Build history of the part. All positions in model axes, mm. A direction names the side the tool comes from. Round coordinates to 2 decimals unless told otherwise and drop trailing zeros. Write each loop counter-clockwise with the first axis right and the second up, starting at its lowest first coordinate (ties: lowest second). Pieces come first, ordered by that corner, then holes.
Item 1: Band-saw the part on C-C, the plane x = -3. Write the cut outline in (y, z), then the cut area to 3 significant figures.
Item 2: Wall check: probe 1 along Y at (x, z) = (1.75, 5.25); probe 2 along Y at (x, z) = (-1, 2); probe 3 along X at (y, z) = (3, -2.25). Give the ranges that are in metal, low to high.
Item 3: Band-saw the part on B-B, the plane x = 0. Write the cut outline in (y, z).
Item 4: 3-axis set-ups, long thin cutter, end or side, ignore diameter. For faces 4 (the cylindrical face through (0, 1.1, 2.7)), 5 (the flat face through (-5.5, 16, 0)): which of +Z, -Z, +X, -X, +Y, -Y reach the whole face in a straight line?
Item 5: Band-saw the part on A-A, the plane y = 4. Write the cut outline in (x, z) (1 decimal).
Item 6: Mould opens along X. For faces 1 (the flat face through (0, 5, 1.7)), 2 (the flat face through (0, 16, -5.5)), 3 (the flat face through (5.5, 16, 0)) say: +X half, -X half, draft (parallel to the pull), parting line (faces both ways), or undercut.
Item 7: Drop flat-ended pins along their axis: pin 1 Ø1 at (x, y) = (-3, 10.5) entering from +Z; pin 2 Ø1 at (x, z) = (1.5, -0.5) entering from -Y; pin 3 Ø1.1 at (y, z) = (3, 0.5) entering from -X. Give the stop position or say it passes through.
Autodesk Inventor part; units mm, degrees
ref_plane "YZ Plane" through (0, 0, 0) normal (1, 0, 0) x (0, 1, 0)
ref_plane "XZ Plane" through (0, 0, 0) normal (0, 1, 0) x (-1, 0, 0)
ref_plane "XY Plane" through (0, 0, 0) normal (0, 0, 1) x (1, 0, 0)
sketch "Sketch1" plane through (0, 0, 0) normal (0, 1, 0) x (-1, 0, 0)
  line L0 (14.5, -14.5) -> (-14.5, -14.5)
  line L1 (-14.5, -14.5) -> (-14.5, 14.5)
  line L2 (-14.5, 14.5) -> (14.5, 14.5)
  line L3 (14.5, 14.5) -> (14.5, -14.5)
  circle A0 centre (0, 0) radius 4
  dimension "d11" = 29
  dimension "d14" = 29
  dimension "d31" = 8
extrude "Extrusion1" add sketch "Sketch1" along normal blind 11.5 contours A0
sketch "Sketch2" plane through (0, 11.5, 0) normal (0, 1, 0) x (1, 0, 0)
  line L0 (-5.5, 5.5) -> (5.5, 5.5)
  line L1 (5.5, 5.5) -> (5.5, -5.5)
  line L2 (5.5, -5.5) -> (-5.5, -5.5)
  line L3 (-5.5, -5.5) -> (-5.5, 5.5)
  line L4 (14.5, 14.5) -> (-14.5, 14.5)
  line L5 (14.5, -14.5) -> (14.5, 14.5)
  line L6 (-14.5, -14.5) -> (14.5, -14.5)
  line L7 (-14.5, 14.5) -> (-14.5, -14.5)
  point P0 (0, 0)
  dimension "d15" = 9
  dimension "d16" = 9
  dimension "d17" = 9
  dimension "d18" = 9
  dimension "d32" = 11
extrude "Extrusion2" add sketch "Sketch2" along normal blind 10 contours L0 L1 L2 L3
sketch "Sketch3" plane through (0, 0, 0) normal (0, -1, 0) x (1, 0, 0)
  line L0 (-0.0005, -0.0003) -> (-0.0005, -1.7003)
  line L1 (-0.0005, -1.7003) -> (2.6995, -1.7003)
  line L2 (2.6995, -1.7003) -> (2.6995, 1.6997)
  line L3 (2.6995, 1.6997) -> (-2.7005, 1.6997)
  line L4 (-2.7005, 1.6997) -> (-2.7005, -1.7003)
  line L5 (-2.7005, -1.7003) -> (-0.0005, -1.7003)
  dimension "d42" = 1.7
  dimension "d43" = 2.7
  dimension "d44" = 3.4
  dimension "d45" = 5.4
extrude "Extrusion3" cut sketch "Sketch3" against normal blind 8.2
sketch "Sketch5" plane through (0, 0, 0) normal (0, -1, 0) x (1, 0, 0)
  circle A0 centre (0, 0) radius 2.7
  dimension "d35" = 5.4
extrude "Extrusion4" cut sketch "Sketch5" against normal blind 2.2
fillet "Fillet1" radius 0.635 4 edges at (2.6995, 4.1, 1.6997) (2.6995, 4.1, -1.7003) (-2.7005, 4.1, -1.7003) (-2.7005, 4.1, 1.6997)
equation "\"d14\" = d11"
equation "\"d16\" = d15"
equation "\"d17\" = d15"
equation "\"d18\" = d15"
equation "\"d42\" = 0.5 * d44"
properties part number "Motor_fit_check"
Results:
1. outline: (0, -2.65) - (11.5, -2.65) - (11.5, -5.5) - (21.5, -5.5) - (21.5, 5.5) - (11.5, 5.5) - (11.5, 2.65) - (0, 2.65) - close
1. area: 171 mm2
2. probe 1: y = 11.5 to 21.5
2. probe 2: y = 2.2 to 21.5
2. probe 3: x = -3.31 to 3.31
3. outline: (0, -4) - (11.5, -4) - (11.5, -5.5) - (21.5, -5.5) - (21.5, 5.5) - (11.5, 5.5) - (11.5, 4) - (0, 4) - (0, 2.7) - (2.2, 2.7) - (2.2, 1.7) - (8.2, 1.7) - (8.2, -1.7) - (2.2, -1.7) - (2.2, -2.7) - (0, -2.7) - close
4. face 4: -Y
4. face 5: +Z, -Z, -X, +Y, -Y
5. outline: circle Ø8 at (0, 0); hole (-2.7, -1.1) arc R0.6 ccw to (-2.1, -1.7) - (2.1, -1.7) arc R0.6 ccw to (2.7, -1.1) - (2.7, 1.1) arc R0.6 ccw to (2.1, 1.7) - (-2.1, 1.7) arc R0.6 ccw to (-2.7, 1.1) - close
6. face 1: undercut
6. face 2: draft
6. face 3: +X half
7. pin 1: stops at z = 3.12
7. pin 2: stops at y = 8.2
7. pin 3: stops at x = -4
